Can you work these out from the model? Positions are in its coordinate system, mm. A direction names the side the tool comes from. Coordinates: 2 decimals unless noted, no trailing zeros. Write each loop counter-clockwise with the first axis right and the second up, starting at its lowest first coordinate (ties: lowest second). Pieces come first, ordered by that corner, then holes. Notation, with made-up numbers: (60, -10) - (85, -10) arc R13 ccw to (85, 0) - close; hole circle Ø4 at (-10, 71.25). An arc over 180 degrees is marked (long way). One line per question, with ' | ' between items. Start each with the question number.
Autodesk Inventor part; units mm, degrees
ref_plane "YZ Plane" through (0, 0, 0) normal (1, 0, 0) x (0, 1, 0)
ref_plane "XZ Plane" through (0, 0, 0) normal (0, 1, 0) x (-1, 0, 0)
ref_plane "XY Plane" through (0, 0, 0) normal (0, 0, 1) x (1, 0, 0)
sketch "Sketch1" plane through (0, 0, 0) normal (0, 0, 1) x (1, 0, 0)
  circle A0 centre (0, 0) radius 5
  circle A1 centre (0, 0) radius 3.175
  dimension "d0" = 10
  dimension "d1" = 6.35
extrude "Extrusion1" add sketch "Sketch1" along normal blind 10
sketch "Sketch2" plane through (0, 0, 10) normal (0, 0, 1) x (1, 0, 0)
  circle A0 centre (0, 0) radius 5
  circle A1 centre (0, 0) radius 6.5
  dimension "d4" = 13
sketch "Sketch4" plane through (0, 0, 0) normal (0, 0, -1) x (-1, 0, 0)
  circle A0 centre (0, 0) radius 6.5
  circle A1 centre (0, 0) radius 5
  dimension "d8" = 13
extrude "Extrusion2" add sketch "Sketch2" against normal blind 2
extrude "Extrusion3" add sketch "Sketch4" against normal blind 2
equation "\"d11\" = d9"
properties part number "spindle"
(1) I'm going to push flat-ended pins straight in: pin 1 (1.5 mm diameter, centred on x = 3, z = 3, fed in from +Y); pin 2 (3 mm diameter, centred on x = -2.5, y = -1, fed in from +Z); pin 3 (1.5 mm diameter, centred on x = -3, z = 1.5, fed in from -Y). Where does each tip first touch, or does it pass through?
(2) If we mould it in two halves opening along Y, with no side actions, what happens to faces 1 (the face through (-0.69, 3.1, 4.93)), 2 (the face through (5.158, -3.955, 0.986)), 3 (the face through (-2, -5, 2))? For each: +Y half, -Y half, draft (parallel to the pull), parting line (faces both ways), or undercut.
(3) If we section it at D-D on y = -5.25: List the corners of the cut face in (x, z) for me.
(4) If I drill on probe 1 along Z at (x, y) = (5, -3.25); probe 2 along Y at (x, z) = (0, 3.5) (3 decimals); probe 3 along X at (y, z) = (2.75, 8.25), over which ranges is the centre line in solid material (lowest first)?
(5) Which directions (+Z, -Z, +X, -X, +Y, -Y) give clear straight access to the entire face, cutting with the end or side of a thin tool? Please do faces 4 (the face through (3, 2, 10)), 5 (the face through (-1.08, 4.88, 4.96)).
(6) If we section it at A-A on x = 0: List the corners of the cut face in (y, z) for me (3 decimals), plus the area to 3 significant figures.
(7) If we section it at C-C on z = 7: List the corners of the cut face in (x, y) for me (3 decimals), plus the area to 3 significant figures.
Values:
1) pin 1: y = 4.47 | pin 2: z = 10 | pin 3: y = -6.1
2) face 1: undercut | face 2: parting line | face 3: draft
3) outline: (-3.83, 0) - (3.83, 0) - (3.83, 2) - (-3.83, 2) - close; (-3.83, 8) - (3.83, 8) - (3.83, 10) - (-3.83, 10) - close
4) probe 1: 0 to 2, 8 to 10 | probe 2: -5 to -3.175, 3.175 to 5 | probe 3: -5.89 to -1.59, 1.59 to 5.89
5) face 4: +Z, +X, -X, +Y, -Y | face 5: none
6) outline: (-6.5, 0) - (-3.175, 0) - (-3.175, 10) - (-6.5, 10) - (-6.5, 8) - (-5, 8) - (-5, 2) - (-6.5, 2) - close; (3.175, 0) - (6.5, 0) - (6.5, 2) - (5, 2) - (5, 8) - (6.5, 8) - (6.5, 10) - (3.175, 10) - close | area: 48.5 mm2
7) outline: circle Ø10 at (0, 0); hole circle Ø6.35 at (0, 0) | area: 46.9 mm2
